```python
from build123d import *

# Parameters (mm, degrees)
BOSS_EXTRUDE2_DEPTH = 304.8
SKETCH3_W           = 12.7
SKETCH3_H           = 10.668
BOSS_EXTRUDE3_DEPTH = 12.192
FILLET1_R           = 0.508
SKETCH4_R           = 4.7625
CUT_EXTRUDE1_DEPTH  = 318.304868037
SKETCH5_W           = 13.208
SKETCH5_H           = 11.176
CUT_EXTRUDE2_DEPTH  = 12.7
FILLET3_R           = 0.381
FILLET4_R           = 0.254


with BuildPart() as part:
    # Sketch2 → Boss-Extrude2 (new body)
    with BuildSketch(Plane(origin=(0, 0, 0), x_dir=(1, 0, 0), z_dir=(0, 1, 0))):
        Polygon((-6.604, 6.096), (6.604, 6.096), (12.7, 0), (6.604, -6.096), (-6.604, -6.096), (-12.7, 0), align=None)
    extrude(amount=BOSS_EXTRUDE2_DEPTH)

    # Sketch3 → Boss-Extrude3 (add)
    with BuildSketch(Plane.XZ):
        Rectangle(SKETCH3_W, SKETCH3_H)
    extrude(amount=BOSS_EXTRUDE3_DEPTH)

    # Fillet1
    fillet1_edges = [part.edges().sort_by_distance(p)[0] for p in [
        (6.35, 0, 0),
        (6.35, -6.096, -5.334),
        (0, 0, 5.334),
        (6.35, -6.096, 5.334),
        (-6.35, 0, 0),
        (-6.35, -6.096, 5.334),
        (0, 0, -5.334),
        (-6.35, -6.096, -5.334),
        (6.35, -12.192, 0),
        (0, -12.192, 5.334),
        (-6.35, -12.192, 0),
        (0, -12.192, -5.334),
    ]]
    fillet(fillet1_edges, radius=FILLET1_R)

    # Sketch4 → Cut-Extrude1 (cut, through all)
    with BuildSketch(Plane(origin=(0, 304.8, 0), x_dir=(1, 0, 0), z_dir=(0, 1, 0))):
        with Locations(Location((0, 0, 0), (0, 0, 270))):
            Circle(SKETCH4_R)
    extrude(amount=-CUT_EXTRUDE1_DEPTH, mode=Mode.SUBTRACT)

    # Sketch5 → Cut-Extrude2 (cut)
    with BuildSketch(Plane(origin=(0, 304.8, 0), x_dir=(1, 0, 0), z_dir=(0, 1, 0))):
        Rectangle(SKETCH5_W, SKETCH5_H)
    extrude(amount=-CUT_EXTRUDE2_DEPTH, mode=Mode.SUBTRACT)

    # Fillet3
    fillet3_edges = [part.edges().sort_by_distance(p)[0] for p in [
        (6.604, 292.1, 0),
        (6.604, 298.45, -5.588),
        (0, 292.1, 5.588),
        (6.604, 298.45, 5.588),
        (-6.604, 292.1, 0),
        (-6.604, 298.45, 5.588),
        (0, 292.1, -5.588),
        (-6.604, 298.45, -5.588),
    ]]
    fillet(fillet3_edges, radius=FILLET3_R)

    # Fillet4
    fillet4_edges = [part.edges().sort_by_distance(p)[0] for p in [
        (0, 304.8, 5.588),
        (-6.604, 304.8, 0),
        (6.492407684, 304.8, -5.476407684),
        (6.492407684, 304.8, 5.476407684),
        (-6.492407684, 304.8, 5.476407684),
        (-6.492407684, 304.8, -5.476407684),
        (0, 304.8, -5.588),
        (6.604, 304.8, 0),
    ]]
    fillet(fillet4_edges, radius=FILLET4_R)


solid = part.part
```
Verification items for the finished model (mm, model axes). A direction names the side the tool comes from. Coordinates: 2 decimals unless noted, no trailing zeros. Order: outer loops, then holes, each group sorted by start corner. A loop starts at its lowest first (then second) coordinate and runs counter-clockwise, first axis right, second up. Notation, with made-up numbers: (36, 28) -> (49, 28) arc R15 cw to (49, 51) -> close; hole circle Ø3 at (52.5, 2.25). An arc over 180 degrees is marked (long way). Put each result on its own line as item: value. Start each with the question number.
1) Tool access check on faces 4 (the flat face through (0, -6, -5.334)), 5 (the flat face through (0, -6, 5.334)), 6 (the flat face through (0, 150, 6.096)), 7 (the flat face through (-6.35, -6, 0)), 8 (the flat face through (0, 299, -5.588)). Record the directions out of +Z, -Z, +X, -X, +Y, -Y that give a thin tool (end or side, any length) a straight path to the whole face; none if there is none.
2) Cross-section at A-A (x = 0). Enter the section's corners in (y, z), plus the area to 3 significant figures.
3) Release check for a two-part mould opening along Z. For faces 1 (the flat face through (-7.5, 0, -0.5)), 2 (the flat face through (9.6, 150.3, -3.1)), 3 (the cylindrical face through (-2.9, 142.08, -3.78)) record: pulls with the +Z half, pulls with the -Z half, needs draft (parallel to the pull), parting line crosses it, or undercut.
4) Go/stop test with flat-tipped pins: pin 1 (3 mm diameter, centred on y = -8.5, z = 0, fed in from -X); pin 2 (3 mm diameter, centred on y = -4.5, z = 0, fed in from +X); pin 3 (1 mm diameter, centred on y = 207, z = -2.5, fed in from +X). Record where each tip stops, or that it passes through.
5) Material ranges on L1, parallel to X at y = 214, z = 0; L2, parallel to Z at x = 0.25, y = 113.5; L3, parallel to Y at x = -10, z = -0.75, recorded low to high.
6) Cross-section at B-B (y = 39.5). Enter the section's corners in (x, z) (1 decimal).
7) Cross-section at C-C (z = 2.5). Enter the section's corners in (x, y).
Geometry check:
1. face 4: -Z, +X, -X, -Y
1. face 5: +Z, +X, -X, -Y
1. face 6: +Z, +X, -X, +Y, -Y
1. face 7: +Z, -Z, -X, -Y
1. face 8: +Y
2. outline: (-12.19, -4.83) arc R0.51 ccw to (-11.68, -5.33) -> (-0.51, -5.33) arc R0.51 cw to (0, -5.84) -> (0, -6.1) -> (304.8, -6.1) -> (304.8, -5.84) arc R0.25 ccw to (304.55, -5.59) -> (292.48, -5.59) arc R0.38 cw to (292.1, -5.21) -> (292.1, -4.76) -> (-12.19, -4.76) -> close; (-12.19, 4.76) -> (292.1, 4.76) -> (292.1, 5.21) arc R0.38 cw to (292.48, 5.59) -> (304.55, 5.59) arc R0.25 ccw to (304.8, 5.84) -> (304.8, 6.1) -> (0, 6.1) -> (0, 5.84) arc R0.51 cw to (-0.51, 5.33) -> (-11.68, 5.33) arc R0.51 ccw to (-12.19, 4.83) -> close
2. area: 806 mm^2
3. face 1: needs draft
3. face 2: pulls with the -Z half
3. face 3: undercut
4. pin 1: stops at x = -6.35
4. pin 2: stops at x = 6.35
4. pin 3: stops at x = 10.7
5. L1: x = -12.7 to -4.76, 4.76 to 12.7
5. L2: z = -6.1 to -4.76, 4.76 to 6.1
5. L3: y = 0 to 304.8
6. outline: (-12.7, 0) -> (-6.6, -6.1) -> (6.6, -6.1) -> (12.7, 0) -> (6.6, 6.1) -> (-6.6, 6.1) -> close; hole circle Ø9.5 at (0, 0)
7. outline: (-10.2, 0) -> (-6.86, 0) arc R0.51 cw to (-6.35, -0.51) -> (-6.35, -11.68) arc R0.51 ccw to (-5.84, -12.19) -> (-4.05, -12.19) -> (-4.05, 292.1) -> (-6.22, 292.1) arc R0.38 cw to (-6.6, 292.48) -> (-6.6, 304.55) arc R0.25 ccw to (-6.86, 304.8) -> (-10.2, 304.8) -> close; (4.05, -12.19) -> (5.84, -12.19) arc R0.51 ccw to (6.35, -11.68) -> (6.35, -0.51) arc R0.51 cw to (6.86, 0) -> (10.2, 0) -> (10.2, 304.8) -> (6.86, 304.8) arc R0.25 ccw to (6.6, 304.55) -> (6.6, 292.48) arc R0.38 cw to (6.22, 292.1) -> (4.05, 292.1) -> close
